Geometry: final body of the model. Coordinates: model frame, mm. A direction names the side the tool comes from. Coordinates: 2 decimals unless noted, no trailing zeros. Loops run counter-clockwise (first coordinate to the right, second up) from the corner with the lowest first, then second, coordinate; pieces in that order, holes last. Notation, with made-up numbers: (64, 13) -> (69, 13) arc R24 ccw to (69, 46) -> close; hole circle Ø1 at (34.25, -12). An arc over 180 degrees is marked (long way). One line per item, written item: value. Start each with the question number.
Item 1: Mould query, pull axis X, two halves, no side actions, for faces 1 (the flat face through (0, -7, -50)), 2 (the flat face through (55, -15, -13)), 3 (the flat face through (-60, -4, 17)). Classes: +X half, -X half, draft (parallel to the pull), parting line (faces both ways), or undercut.
Item 2: Set-up query: faces 4 (the flat face through (55, -15, 20)), 5 (the flat face through (50, -15, -8)), 6 (the flat face through (-20, -7, -11)). Return all of +Z, -Z, +X, -X, +Y, -Y with unobstructed straight access to the full face (end or side cutting, diameter ignored); none if empty.
Item 3: Ray query, probe 1 along Z at (x, y) = (-16, -11.5); probe 2 along X at (y, z) = (-6.75, 12.5); probe 3 along Z at (x, y) = (-11.5, -2.75). Return the intervals inside material, ascending. Write a range as from..to.
Item 4: Section query D-D on x = 4.5. Return loops of the section in (y, z), then the cut area to 3 significant figures.
Item 5: Contact query for flat-ended pins moving along their axis: pin 1 Ø5 at (x, y) = (-53.5, -20) entering from -Z; pin 2 Ø10 at (y, z) = (-16, -55) entering from -X; pin 3 Ø1 at (y, z) = (-10.5, -40.5) entering from +X. Output: stop coordinate, or through.
Item 6: Section query A-A on y = -7.5. Return loops of the section in (x, z), then the cut area to 3 significant figures.
Item 7: Section query C-C on y = -22.25. Return loops of the section in (x, z), then the cut area to 3 significant figures.
Item 8: Section query B-B on z = -21. Return loops of the section in (x, y), then the cut area to 3 significant figures.
from build123d import *

# Parameters (mm, degrees)
F0_W     = 120
F0_H     = 150
F1_DEPTH = 5
F2_W     = 40
F2_H     = 80
F3_DEPTH = 5.001
F4_W     = 10
F4_H     = 40
F4_H_2   = 10
F5_DEPTH = 20
F6_W     = 40
F6_H     = 10
F7_DEPTH = 10


with BuildPart() as f1:
    # F0 (on Front) → F1 (new body)
    with BuildSketch(Plane.XZ):
        with Locations((0, -15)):
            Rectangle(F0_W, F0_H)
    extrude(amount=F1_DEPTH)

    # F2 (on face) → F3 (cut, through all)
    with BuildSketch(Plane.XZ.offset(5)):
        with Locations((0, -10)):
            Rectangle(F2_W, F2_H)
    extrude(amount=-F3_DEPTH, mode=Mode.SUBTRACT)

    # F4 (on face) → F5 (join)
    with BuildSketch(Plane.XZ.offset(5)):
        with Locations((-55, 40)):
            Rectangle(F4_W, F4_H)
        with Locations((-55, -8)):
            Rectangle(F4_W, F4_H_2)
        with Locations((55, 40)):
            Rectangle(F4_W, F4_H)
        with Locations((55, -8)):
            Rectangle(F4_W, F4_H_2)
    extrude(amount=F5_DEPTH)

    # F6 (on face) → F7 (join)
    with BuildSketch(Plane.XZ.offset(5)):
        with Locations((0, 35)):
            Rectangle(F6_W, F6_H)
        Polygon((-20, -50), (-20, 30), (-20, 40), (-25, 40), (-25, -60), (-20, -60), align=None)
        Polygon((20, 40), (20, 30), (20, -50), (20, -60), (25, -60), (25, 40), align=None)
        with Locations((0, -55)):
            Rectangle(F6_W, F6_H)
    extrude(amount=F7_DEPTH)


solid = f1.part
Reply:
1. face 1: undercut
1. face 2: draft
1. face 3: -X half
2. face 4: +X, -Y
2. face 5: +Z, -Z, -Y
2. face 6: +Y, -Y
3. probe 1: z = -60..-50, 30..40
3. probe 2: x = -25..-20, 20..25
3. probe 3: z = -90..-50, 30..60
4. outline: (-15, -60) -> (-5, -60) -> (-5, -90) -> (0, -90) -> (0, -50) -> (-15, -50) -> close; (-15, 30) -> (0, 30) -> (0, 60) -> (-5, 60) -> (-5, 40) -> (-15, 40) -> close
4. area: 550 mm²
5. pin 1: stops at z = -13
5. pin 2: stops at x = -25
5. pin 3: stops at x = 25
6. outline: (-60, -13) -> (-50, -13) -> (-50, -3) -> (-60, -3) -> close; (-60, 20) -> (-50, 20) -> (-50, 60) -> (-60, 60) -> close; (-25, -60) -> (25, -60) -> (25, 40) -> (-25, 40) -> close; (50, -13) -> (60, -13) -> (60, -3) -> (50, -3) -> close; (50, 20) -> (60, 20) -> (60, 60) -> (50, 60) -> close; hole (-20, -50) -> (20, -50) -> (20, 30) -> (-20, 30) -> close
6. area: 2,800 mm²
7. outline: (-60, -13) -> (-50, -13) -> (-50, -3) -> (-60, -3) -> close; (-60, 20) -> (-50, 20) -> (-50, 60) -> (-60, 60) -> close; (50, -13) -> (60, -13) -> (60, -3) -> (50, -3) -> close; (50, 20) -> (60, 20) -> (60, 60) -> (50, 60) -> close
7. area: 1,000 mm²
8. outline: (-60, -5) -> (-25, -5) -> (-25, -15) -> (-20, -15) -> (-20, 0) -> (-60, 0) -> close; (20, -15) -> (25, -15) -> (25, -5) -> (60, -5) -> (60, 0) -> (20, 0) -> close
8. area: 500 mm²
